Answer from the drawing. Dimensions are ordinates in mm from the lowest x, y and z of the part. A direction names the side the tool comes from. Give positions to 0.01 mm unless a question says otherwise; leave off trailing zeros. Write each loop counter-clockwise with the first axis right and the second up, starting at its lowest first coordinate (ties: lowest second). Pieces come first, ordered by that corner, then holes.
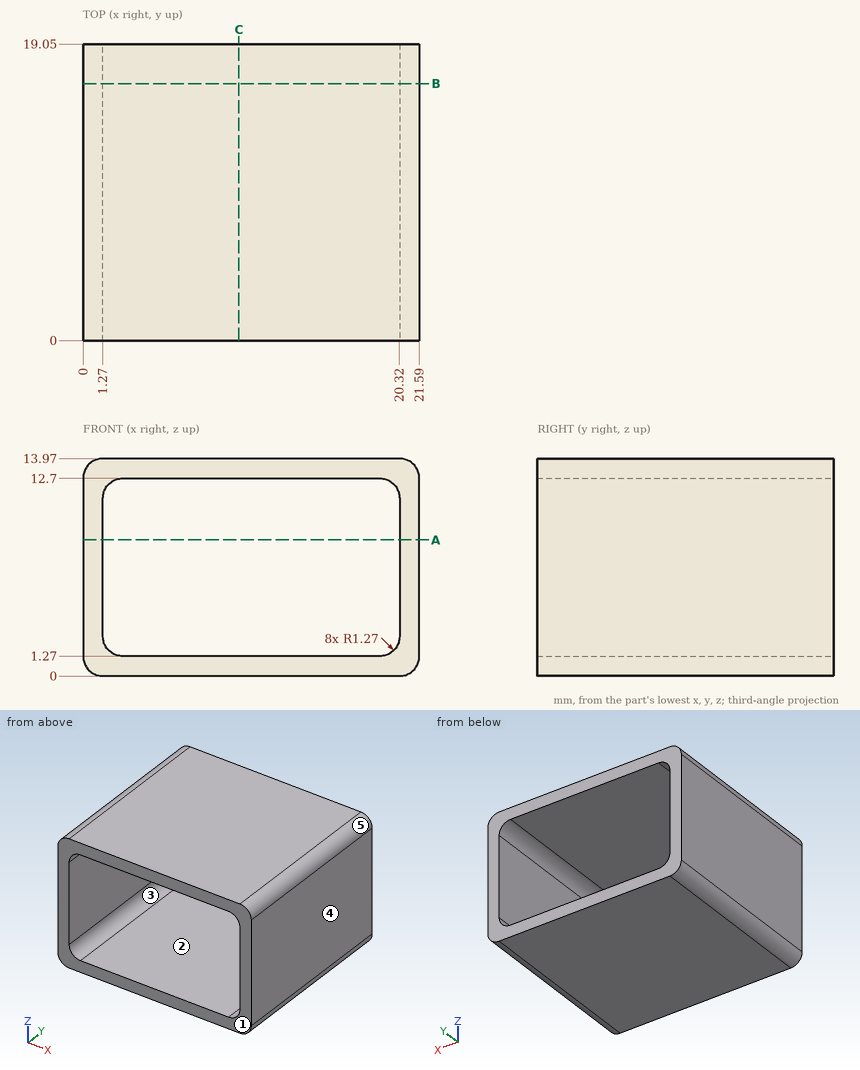
Item 1: Section B-B (y = 16.5) is taken. Write down the section's boundary in (x, z).
Result set:
outline: (0, 1.27) arc R1.27 ccw to (1.27, 0) - (20.32, 0) arc R1.27 ccw to (21.59, 1.27) - (21.59, 12.7) arc R1.27 ccw to (20.32, 13.97) - (1.27, 13.97) arc R1.27 ccw to (0, 12.7) - close; hole (1.27, 2.54) arc R1.27 ccw to (2.54, 1.27) - (19.05, 1.27) arc R1.27 ccw to (20.32, 2.54) - (20.32, 11.43) arc R1.27 ccw to (19.05, 12.7) - (2.54, 12.7) arc R1.27 ccw to (1.27, 11.43) - close
Item 2: Determine the mould class of the marked faces 3, 4 and 5 for opening direction Z: pulls with the +Z half, pulls with the -Z half, needs draft (parallel to the pull), parting line crosses it, or undercut.
Result set:
face 3: undercut
face 4: needs draft
face 5: pulls with the +Z half
Item 3: Section C-C (x = 10) is taken. Write down the section's boundary in (y, z), and give its area (3 significant figures).
Result set:
outline: (0, 0) - (19.05, 0) - (19.05, 1.27) - (0, 1.27) - close; (0, 12.7) - (19.05, 12.7) - (19.05, 13.97) - (0, 13.97) - close
area: 48.4 mm2
Item 4: Section A-A (z = 8.75) is taken. Write down the section's boundary in (x, y).
Result set:
outline: (0, 0) - (1.27, 0) - (1.27, 19.05) - (0, 19.05) - close; (20.32, 0) - (21.59, 0) - (21.59, 19.05) - (20.32, 19.05) - close
Item 5: Which of the six approach directions +Z, -Z, +X, -X, +Y, -Y give full straight-line access (tool end or side, diameter ignored) to the marked faces 1 and 2?
Result set:
face 1: +Z, -Z, +X, -X, -Y
face 2: +Y, -Y
Item 6: Find the intervals of material crossed by line 1 along X through (y, z) = (14, 2.75); line 2 along Z through (x, y) = (4, 12.75); line 3 along Z through (x, y) = (19.5, 13), in increasing order.
Result set:
line 1: x = 0 to 1.27, 20.32 to 21.59
line 2: z = 0 to 1.27, 12.7 to 13.97
line 3: z = 0 to 1.35, 12.62 to 13.97
